from build123d import *

# Parameters (mm, degrees)
SKETCH1_R           = 1.925
BOSS_EXTRUDE1_DEPTH = 2.54
SKETCH2_W           = 48.26
SKETCH2_H           = 20.066
BOSS_EXTRUDE2_DEPTH = 9.398
BOSS_EXTRUDE3_DEPTH = 25.4
SKETCH4_R           = 8.5
CUT_EXTRUDE1_DEPTH  = 2


with BuildPart() as part:
    # Sketch1 → Boss-Extrude1 (new body)
    with BuildSketch(Plane(origin=(0, 0, 0), x_dir=(1, 0, 0), z_dir=(0, 1, 0))):
        with BuildLine():
            Line((-24.13, 10.033), (-20.724, 10.033))
            ThreePointArc((-20.724, 10.033), (-18.602679656, 10.911679656), (-17.724, 13.033))
            Line((-17.724, 13.033), (-17.724, 13.716))
            ThreePointArc((-17.724, 13.716), (-14.224, 17.216), (-10.724, 13.716))
            Line((-10.724, 13.716), (-10.724, 13.033))
            ThreePointArc((-10.724, 13.033), (-9.845320344, 10.911679656), (-7.724, 10.033))
            Line((-7.724, 10.033), (7.724, 10.033))
            ThreePointArc((7.724, 10.033), (9.845320344, 10.911679656), (10.724, 13.033))
            Line((10.724, 13.033), (10.724, 13.716))
            ThreePointArc((10.724, 13.716), (14.224, 17.216), (17.724, 13.716))
            Line((17.724, 13.716), (17.724, 13.033))
            ThreePointArc((17.724, 13.033), (18.602679656, 10.911679656), (20.724, 10.033))
            Line((20.724, 10.033), (24.13, 10.033))
            Line((24.13, 10.033), (24.13, -10.033))
            Line((24.13, -10.033), (20.724, -10.033))
            ThreePointArc((20.724, -10.033), (18.602679656, -10.911679656), (17.724, -13.033))
            Line((17.724, -13.033), (17.724, -13.716))
            ThreePointArc((17.724, -13.716), (14.224, -17.216), (10.724, -13.716))
            Line((10.724, -13.716), (10.724, -13.033))
            ThreePointArc((10.724, -13.033), (9.845320344, -10.911679656), (7.724, -10.033))
            Line((7.724, -10.033), (-7.724, -10.033))
            ThreePointArc((-7.724, -10.033), (-9.845320344, -10.911679656), (-10.724, -13.033))
            Line((-10.724, -13.033), (-10.724, -13.716))
            ThreePointArc((-10.724, -13.716), (-14.224, -17.216), (-17.724, -13.716))
            Line((-17.724, -13.716), (-17.724, -13.033))
            ThreePointArc((-17.724, -13.033), (-18.602679656, -10.911679656), (-20.724, -10.033))
            Line((-20.724, -10.033), (-24.13, -10.033))
            Line((-24.13, -10.033), (-24.13, 10.033))
        make_face()
        with Locations(Location((-14.224, 13.716, 0), (0, 0, 270))):
            Circle(SKETCH1_R, mode=Mode.SUBTRACT)
        with Locations(Location((-14.224, -13.716, 0), (0, 0, 90))):
            Circle(SKETCH1_R, mode=Mode.SUBTRACT)
        with Locations(Location((14.224, -13.716, 0), (0, 0, 270))):
            Circle(SKETCH1_R, mode=Mode.SUBTRACT)
        with Locations(Location((14.224, 13.716, 0), (0, 0, 90))):
            Circle(SKETCH1_R, mode=Mode.SUBTRACT)
    extrude(amount=BOSS_EXTRUDE1_DEPTH)

    # Sketch2 → Boss-Extrude2 (add)
    with BuildSketch(Plane(origin=(0, 2.54, 0), x_dir=(1, 0, 0), z_dir=(0, 1, 0))):
        Rectangle(SKETCH2_W, SKETCH2_H)
    extrude(amount=BOSS_EXTRUDE2_DEPTH)

    # Sketch3 → Boss-Extrude3 (add)
    with BuildSketch(Plane(origin=(0, 11.938, 0), x_dir=(1, 0, 0), z_dir=(0, 1, 0))):
        with BuildLine():
            Line((-3.808215378, 5), (3.808215378, 5))
            ThreePointArc((3.808215378, 5), (5.126464602, 5.305149544), (6.176538394, 6.158520678))
            ThreePointArc((6.176538394, 6.158520678), (24.13, 0), (6.176538394, -6.158520678))
            ThreePointArc((6.176538394, -6.158520678), (5.126464602, -5.305149544), (3.808215378, -5))
            Line((3.808215378, -5), (-3.808215378, -5))
            ThreePointArc((-3.808215378, -5), (-5.126464602, -5.305149544), (-6.176538394, -6.158520678))
            ThreePointArc((-6.176538394, -6.158520678), (-24.13, 0), (-6.176538394, 6.158520678))
            ThreePointArc((-6.176538394, 6.158520678), (-5.126464602, 5.305149544), (-3.808215378, 5))
        make_face()
    extrude(amount=BOSS_EXTRUDE3_DEPTH)

    # Sketch4 → Cut-Extrude1 (cut)
    with BuildSketch(Plane(origin=(0, 37.338, 0), x_dir=(1, 0, 0), z_dir=(0, 1, 0))):
        with Locations(Location((14.097, 0, 0), (0, 0, 270))):
            Circle(SKETCH4_R)
        with Locations(Location((-14.097, 0, 0), (0, 0, 90))):
            Circle(SKETCH4_R)
    extrude(amount=-CUT_EXTRUDE1_DEPTH, mode=Mode.SUBTRACT)


solid = part.part
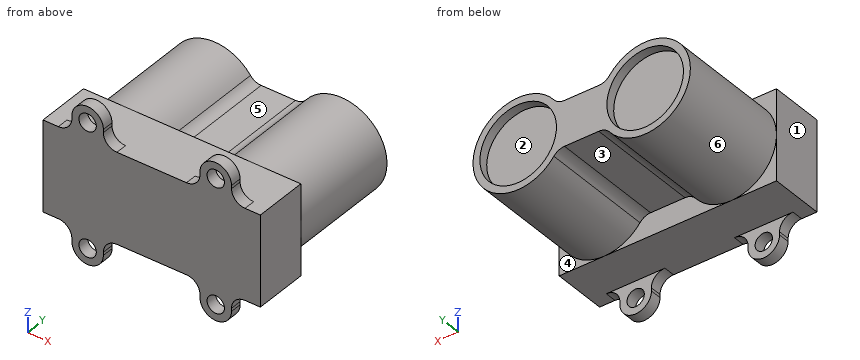
Geometry check sheet. Reference: the model listing, model coordinates, mm. Face numbers are marked on the shaded views. A direction names the side the tool comes from. Round coordinates to 2 decimals unless told otherwise and drop trailing zeros. Order: outer loops, then holes, each group sorted by start corner. A loop starts at its lowest first (then second) coordinate and runs counter-clockwise, first axis right, second up. Notation, with made-up numbers: M 78.25,41.25 L 108.25,41.25 A14 ccw 108.25,49.25 Z; hole C 88.5,-27.5 d10. An arc over 180 degrees is marked long. Answer in a Markdown table with one row per item. Add a question column.
Item 1: Set-up check for the marked faces 4, 5 and 6: record each of +Z, -Z, +X, -X, +Y, -Y from which the full face is reachable in a straight line by a thin tool's end or side.
Item 2: Sectioned sample at D-D, the plane x = -2. Enter the section's corners in (y, z).
Item 3: Sectioned sample at A-A, the plane y = 32.5. Enter the section's corners in (x, z), plus the area to 3 significant figures.
Item 4: Sectioned sample at B-B, the plane x = 9. Enter the section's corners in (y, z).
Item 5: Depth check by flat-ended pin: pin 1 Ø1 at (x, z) = (18, -13.5) entering from +Y; pin 2 Ø4 at (x, z) = (1, 7.5) entering from +Y; pin 3 Ø1 at (y, z) = (27.5, 6.5) entering from -X. Enter the tip coordinate at first touch or a pass-through.
Item 6: Material ranges on L1, parallel to X at y = 36, z = 0; L2, parallel to Z at x = 17, y = 11.5; L3, parallel to Y at x = 10, z = 5, recorded low to high. Write a range as [from, to].
Item 7: Draft check along Z on the marked faces 1, 2 and 3. Enter one of: released by +Z, released by -Z, zero draft, split by the parting line, or undercut.
Item 8: Sectioned sample at C-C, the plane z = 3. Enter the section's corners in (x, y), plus the area to 3 significant figures.
Filled in:
| question | item | result |
|---|---|---|
| 1 | face 4 | -Z, +X, +Y |
| 1 | face 5 | +Z, +Y |
| 1 | face 6 | +Y |
| 2 | outline | M 0,-10.03 L 11.94,-10.03 L 11.94,-5 L 37.34,-5 L 37.34,5 L 11.94,5 L 11.94,10.03 L 0,10.03 Z |
| 3 | outline | M -6.18,-6.16 A3 cw -3.81,-5 L 3.81,-5 A3 cw 6.18,-6.16 A10.03 ccw long 6.18,6.16 A3 cw 3.81,5 L -3.81,5 A3 cw -6.18,6.16 A10.03 ccw long Z |
| 3 | area | 724 mm² |
| 4 | outline | M 0,-10.32 L 2.54,-10.32 L 2.54,-10.03 L 11.94,-10.03 L 11.94,-8.64 L 37.34,-8.64 L 37.34,-6.8 L 35.34,-6.8 L 35.34,6.8 L 37.34,6.8 L 37.34,8.64 L 11.94,8.64 L 11.94,10.03 L 2.54,10.03 L 2.54,10.32 L 0,10.32 Z |
| 5 | pin 1 | stops at y = 2.54 |
| 5 | pin 2 | stops at y = 11.94 |
| 5 | pin 3 | stops at x = -22.14 |
| 6 | L1 | x = [-24.13, -22.6], [-5.6, 5.6], [22.6, 24.13] |
| 6 | L2 | z = [-10.03, 10.03] |
| 6 | L3 | y = [0, 35.34] |
| 7 | face 1 | zero draft |
| 7 | face 2 | undercut |
| 7 | face 3 | released by -Z |
| 8 | outline | M -24.13,0 L 24.13,0 L 24.13,11.94 L 23.67,11.94 L 23.67,37.34 L 22.05,37.34 L 22.05,35.34 L 6.14,35.34 L 6.14,37.34 L -6.14,37.34 L -6.14,35.34 L -22.05,35.34 L -22.05,37.34 L -23.67,37.34 L -23.67,11.94 L -24.13,11.94 Z |
| 8 | area | 1,710 mm² |
